Could you check a few things on this drawing? It's one solid part, dimensions in mm from its lowest x, y, z. Round coordinates to 2 decimals unless told otherwise and drop trailing zeros. Write each loop counter-clockwise with the first axis right and the second up, starting at its lowest first coordinate (ties: lowest second). Pieces come first, ordered by that corner, then holes. Notation, with made-up numbers: (-34, 62.5) -> (-1, 62.5) arc R10 cw to (-1, 80.5) -> close; hole circle Ø9 at (39.5, 8). An arc over 180 degrees is marked (long way). Answer in a Markdown table with one row per item. Add a question column.
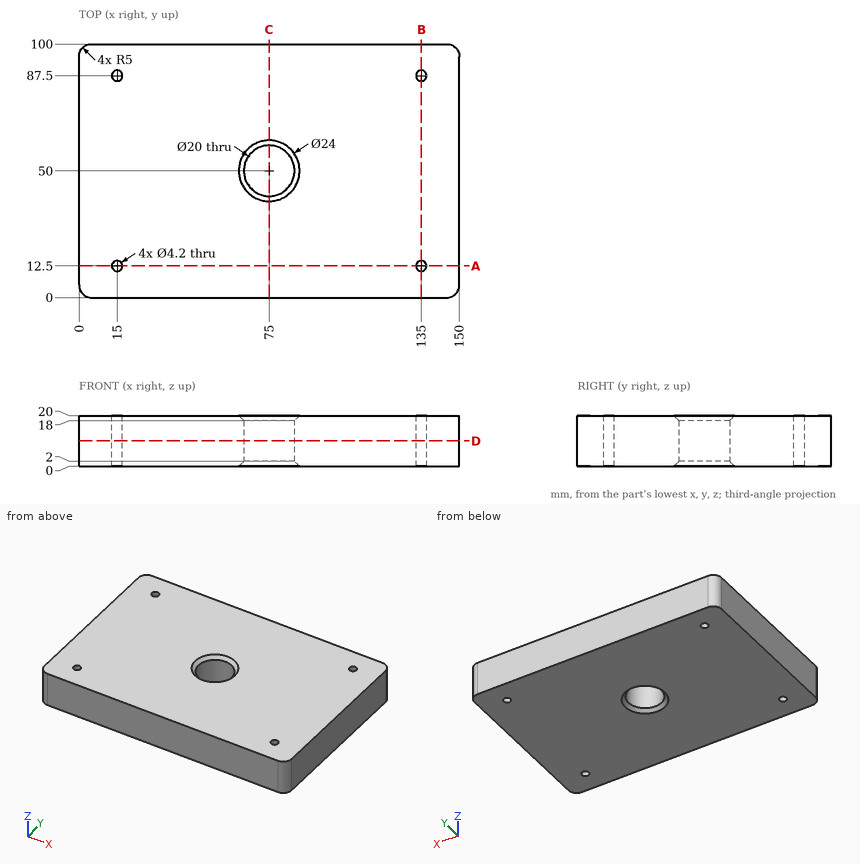
Item 1: If we section it at B-B on x = 135: Please give me the cut outline in (y, z), then the cut area to 3 significant figures.
Item 2: For P1, Ø23, axis at x = 75, y = 50, coming from the -Z side, with a flat end and sliding along its axis, tell me the tip position at first contact or that it passes through.
Item 3: If we section it at A-A on y = 12.5: Please give me the cut outline in (x, z), then the cut area to 3 significant figures.
Item 4: I need wall thicknesses on line 1 along X through (y, z) = (87.5, 11); line 2 along Y through (x, z) = (135, 13.5); line 3 along Y through (x, z) = (75, 13.25). Which ranges of each line are inside material? Lowest first, please. Write a range as from..to.
Item 5: If we section it at C-C on x = 75: Please give me the cut outline in (y, z).
Item 6: If we section it at D-D on z = 10: Please give me the cut outline in (x, y).
Results list:
| question | item | result |
|---|---|---|
| 1 | outline | (0, 0) -> (10.4, 0) -> (10.4, 20) -> (0, 20) -> close; (14.6, 0) -> (85.4, 0) -> (85.4, 20) -> (14.6, 20) -> close; (89.6, 0) -> (100, 0) -> (100, 20) -> (89.6, 20) -> close |
| 1 | area | 1,830 mm² |
| 2 | P1 | z = 0.5 |
| 3 | outline | (0, 0) -> (12.9, 0) -> (12.9, 20) -> (0, 20) -> close; (17.1, 0) -> (132.9, 0) -> (132.9, 20) -> (17.1, 20) -> close; (137.1, 0) -> (150, 0) -> (150, 20) -> (137.1, 20) -> close |
| 3 | area | 2,830 mm² |
| 4 | line 1 | 0..12.9, 17.1..132.9, 137.1..150 |
| 4 | line 2 | 0..10.4, 14.6..85.4, 89.6..100 |
| 4 | line 3 | 0..40, 60..100 |
| 5 | outline | (0, 0) -> (38, 0) -> (40, 2) -> (40, 18) -> (38, 20) -> (0, 20) -> close; (60, 2) -> (62, 0) -> (100, 0) -> (100, 20) -> (62, 20) -> (60, 18) -> close |
| 6 | outline | (0, 5) arc R5 ccw to (5, 0) -> (145, 0) arc R5 ccw to (150, 5) -> (150, 95) arc R5 ccw to (145, 100) -> (5, 100) arc R5 ccw to (0, 95) -> close; hole circle Ø4.2 at (15, 12.5); hole circle Ø4.2 at (15, 87.5); hole circle Ø20 at (75, 50); hole circle Ø4.2 at (135, 12.5); hole circle Ø4.2 at (135, 87.5) |
